from build123d import *
from OCP.BRepFilletAPI import BRepFilletAPI_MakeChamfer

# Parameters (mm, degrees)
CROQUIS1_W              = 16
CROQUIS1_H              = 65
CROQUIS1_W_2            = 60.56813556
CROQUIS1_H_2            = 14.096609531
SALIENTE_EXTRUIR1_DEPTH = 50
CROQUIS3_W              = 16
CROQUIS3_H              = 3
CROQUIS3_W_2            = 3.053388568
CROQUIS3_H_2            = 16.41437111
CROQUIS3_W_3            = 3.044949639
CROQUIS3_H_3            = 14.096609531
CROQUIS3_W_4            = 3.024386733
SALIENTE_EXTRUIR2_DEPTH = 18
CHAFL_N2_SIZE           = 3
CHAFL_N2_SIZE2          = 1.732050808
CHAFL_N3_SIZE           = 5.196152423
CHAFL_N3_SIZE_2         = 3


with BuildPart() as part:
    # Croquis1 → Saliente-Extruir1 (new body)
    with BuildSketch(Plane.XY):
        with BuildLine():
            Line((-85, 0), (-85, -65))
            ThreePointArc((-85, -65), (-79.142135624, -79.142135624), (-65, -85))
            Line((-65, -85), (65, -85))
            ThreePointArc((65, -85), (79.142135624, -79.142135624), (85, -65))
            Line((85, -65), (85, 0))
            ThreePointArc((85, 0), (0, 85), (-85, 0))
        make_face()
        with Locations((75, -31.476837664)):
            Rectangle(CROQUIS1_W, CROQUIS1_H, mode=Mode.SUBTRACT)
        with BuildLine():
            Line((-65, -65), (65, -65))
            Line((65, -65), (65, 0))
            ThreePointArc((65, 0), (0, 65), (-65, 0))
            Line((-65, 0), (-65, -65))
        make_face(mode=Mode.SUBTRACT)
        with Locations((-75, -31.476837664)):
            Rectangle(CROQUIS1_W, CROQUIS1_H, mode=Mode.SUBTRACT)
        with BuildLine():
            Line((3.510152615, 83.023277843), (3.510152615, 66.83939974))
            ThreePointArc((3.510152615, 66.83939974), (47.145709065, 47.509037517), (66.810483413, 4.023162336))
            Line((66.810483413, 4.023162336), (83, 4.023162336))
            ThreePointArc((83, 4.023162336), (58.576925397, 58.940051292), (3.510152615, 83.023277843))
        make_face(mode=Mode.SUBTRACT)
        with BuildLine():
            Line((-66.810483413, 4.023162336), (-83, 4.023162336))
            ThreePointArc((-83, 4.023162336), (-58.576925397, 58.940051292), (-3.510152615, 83.023277843))
            Line((-3.510152615, 83.023277843), (-3.510152615, 66.83939974))
            ThreePointArc((-3.510152615, 66.83939974), (-47.145709065, 47.509037517), (-66.810483413, 4.023162336))
        make_face(mode=Mode.SUBTRACT)
        with BuildLine():
            Line((-81.096609531, -66.976837664), (-34.71593222, -66.976837664))
            Line((-34.71593222, -66.976837664), (-34.71593222, -81.073447195))
            Line((-34.71593222, -81.073447195), (-67, -81.073447195))
            ThreePointArc((-67, -81.073447195), (-76.967808191, -76.944645855), (-81.096609531, -66.976837664))
        make_face(mode=Mode.SUBTRACT)
        with BuildLine():
            Line((67, -81.073447195), (34.71593222, -81.073447195))
            Line((34.71593222, -81.073447195), (34.71593222, -66.976837664))
            Line((34.71593222, -66.976837664), (81.096609531, -66.976837664))
            ThreePointArc((81.096609531, -66.976837664), (76.967808191, -76.944645855), (67, -81.073447195))
        make_face(mode=Mode.SUBTRACT)
        with Locations((0, -74.025142429)):
            Rectangle(CROQUIS1_W_2, CROQUIS1_H_2, mode=Mode.SUBTRACT)
    extrude(amount=SALIENTE_EXTRUIR1_DEPTH)

    # Croquis3 → Saliente-Extruir2 (add)
    with BuildSketch(Plane.XY.offset(40)):
        with Locations((-75, -0.476837664)):
            Rectangle(CROQUIS3_W, CROQUIS3_H)
        with Locations((-75, -62.476837664)):
            Rectangle(CROQUIS3_W, CROQUIS3_H)
        with Locations((75, -62.476837664)):
            Rectangle(CROQUIS3_W, CROQUIS3_H)
        with Locations((75, -0.476837664)):
            Rectangle(CROQUIS3_W, CROQUIS3_H)
        with Locations((-5.036846899, 74.816092288)):
            Rectangle(CROQUIS3_W_2, CROQUIS3_H_2)
        with Locations((5.036846899, 74.816092288)):
            Rectangle(CROQUIS3_W_2, CROQUIS3_H_2)
        with Locations((-28.761592961, -74.025142429)):
            Rectangle(CROQUIS3_W_3, CROQUIS3_H_3)
        with Locations((28.771874414, -74.025142429)):
            Rectangle(CROQUIS3_W_4, CROQUIS3_H_3)
    extrude(amount=SALIENTE_EXTRUIR2_DEPTH)

    # Chaflán2: one chamfer whose edges measure the first distance from different faces: ONE call of the kernel's chamfer builder (chamfer() names one face for all edges)
    chafl_n2_edges_1 = [part.edges().sort_by_distance(p)[0] for p in [
        (-75, 1.023162336, 58),
    ]]
    chafl_n2_side_1 = [part.faces().sort_by_distance(p)[0] for p in [
        (-75, 1.023162336, 54),
    ]]
    chafl_n2_edges_2 = [part.edges().sort_by_distance(p)[0] for p in [
        (-75, -63.976837664, 58),
    ]]
    chafl_n2_side_2 = [part.faces().sort_by_distance(p)[0] for p in [
        (-75, -63.976837664, 54),
    ]]
    chafl_n2_edges_3 = [part.edges().sort_by_distance(p)[0] for p in [
        (75, -63.976837664, 58),
    ]]
    chafl_n2_side_3 = [part.faces().sort_by_distance(p)[0] for p in [
        (75, -63.976837664, 54),
    ]]
    chafl_n2_edges_4 = [part.edges().sort_by_distance(p)[0] for p in [
        (75, 1.023162336, 58),
    ]]
    chafl_n2_side_4 = [part.faces().sort_by_distance(p)[0] for p in [
        (75, 1.023162336, 54),
    ]]
    chafl_n2_edges_5 = [part.edges().sort_by_distance(p)[0] for p in [
        (-3.510152615, 74.816092288, 58),
    ]]
    chafl_n2_side_5 = [part.faces().sort_by_distance(p)[0] for p in [
        (-3.510152615, 74.816092288, 54),
    ]]
    chafl_n2_edges_6 = [part.edges().sort_by_distance(p)[0] for p in [
        (3.510152615, 74.816092288, 58),
    ]]
    chafl_n2_side_6 = [part.faces().sort_by_distance(p)[0] for p in [
        (3.510152615, 74.816092288, 54),
    ]]
    chafl_n2_edges_7 = [part.edges().sort_by_distance(p)[0] for p in [
        (-30.28406778, -74.025142429, 58),
    ]]
    chafl_n2_side_7 = [part.faces().sort_by_distance(p)[0] for p in [
        (-30.28406778, -74.025142429, 54),
    ]]
    chafl_n2_edges_8 = [part.edges().sort_by_distance(p)[0] for p in [
        (30.28406778, -74.025142429, 58),
    ]]
    chafl_n2_side_8 = [part.faces().sort_by_distance(p)[0] for p in [
        (30.28406778, -74.025142429, 54),
    ]]
    chafl_n2 = BRepFilletAPI_MakeChamfer(part.part.solid().wrapped)
    for e in chafl_n2_edges_1:
        chafl_n2.Add(CHAFL_N2_SIZE, CHAFL_N2_SIZE2, e.wrapped, chafl_n2_side_1[0].wrapped)  # the first distance lies on this face
    for e in chafl_n2_edges_2:
        chafl_n2.Add(CHAFL_N2_SIZE, CHAFL_N2_SIZE2, e.wrapped, chafl_n2_side_2[0].wrapped)  # the first distance lies on this face
    for e in chafl_n2_edges_3:
        chafl_n2.Add(CHAFL_N2_SIZE, CHAFL_N2_SIZE2, e.wrapped, chafl_n2_side_3[0].wrapped)  # the first distance lies on this face
    for e in chafl_n2_edges_4:
        chafl_n2.Add(CHAFL_N2_SIZE, CHAFL_N2_SIZE2, e.wrapped, chafl_n2_side_4[0].wrapped)  # the first distance lies on this face
    for e in chafl_n2_edges_5:
        chafl_n2.Add(CHAFL_N2_SIZE, CHAFL_N2_SIZE2, e.wrapped, chafl_n2_side_5[0].wrapped)  # the first distance lies on this face
    for e in chafl_n2_edges_6:
        chafl_n2.Add(CHAFL_N2_SIZE, CHAFL_N2_SIZE2, e.wrapped, chafl_n2_side_6[0].wrapped)  # the first distance lies on this face
    for e in chafl_n2_edges_7:
        chafl_n2.Add(CHAFL_N2_SIZE, CHAFL_N2_SIZE2, e.wrapped, chafl_n2_side_7[0].wrapped)  # the first distance lies on this face
    for e in chafl_n2_edges_8:
        chafl_n2.Add(CHAFL_N2_SIZE, CHAFL_N2_SIZE2, e.wrapped, chafl_n2_side_8[0].wrapped)  # the first distance lies on this face
    add(Compound.cast(chafl_n2.Shape()), mode=Mode.REPLACE)

    # Chaflán3
    chafl_n3_edges_1 = [part.edges().sort_by_distance(p)[0] for p in [
        (75, -60.976837664, 40),
    ]]
    chafl_n3_side_1 = [part.faces().sort_by_distance(p)[0] for p in [
        (75, -60.976837664, 40.06),
    ]]
    chafl_n3_edges_2 = [part.edges().sort_by_distance(p)[0] for p in [
        (75, -1.976837664, 40),
    ]]
    chafl_n3_side_2 = [part.faces().sort_by_distance(p)[0] for p in [
        (75, -1.976837664, 40.06),
    ]]
    chafl_n3_edges_3 = [part.edges().sort_by_distance(p)[0] for p in [
        (27.259681047, -74.025142429, 40),
    ]]
    chafl_n3_side_3 = [part.faces().sort_by_distance(p)[0] for p in [
        (27.319681047, -74.025142429, 40),
    ]]
    chafl_n3_edges_4 = [part.edges().sort_by_distance(p)[0] for p in [
        (-27.239118141, -74.025142429, 40),
    ]]
    chafl_n3_side_4 = [part.faces().sort_by_distance(p)[0] for p in [
        (-27.239118141, -74.025142429, 40.06),
    ]]
    chafl_n3_edges_5 = [part.edges().sort_by_distance(p)[0] for p in [
        (-75, -60.976837664, 40),
    ]]
    chafl_n3_side_5 = [part.faces().sort_by_distance(p)[0] for p in [
        (-75, -60.976837664, 40.06),
    ]]
    chafl_n3_edges_6 = [part.edges().sort_by_distance(p)[0] for p in [
        (-75, -1.976837664, 40),
    ]]
    chafl_n3_side_6 = [part.faces().sort_by_distance(p)[0] for p in [
        (-75, -1.976837664, 40.06),
    ]]
    chafl_n3_edges_7 = [part.edges().sort_by_distance(p)[0] for p in [
        (-6.563541183, 74.72336741, 40),
    ]]
    chafl_n3_side_7 = [part.faces().sort_by_distance(p)[0] for p in [
        (-6.563541183, 74.72336741, 40.06),
    ]]
    chafl_n3_edges_8 = [part.edges().sort_by_distance(p)[0] for p in [
        (6.563541183, 74.72336741, 40),
    ]]
    chafl_n3_side_8 = [part.faces().sort_by_distance(p)[0] for p in [
        (6.563541183, 74.72336741, 40.06),
    ]]
    chafl_n3 = BRepFilletAPI_MakeChamfer(part.part.solid().wrapped)
    for e in chafl_n3_edges_1:
        chafl_n3.Add(CHAFL_N3_SIZE - 0.0001, CHAFL_N3_SIZE_2 - 0.0001, e.wrapped, chafl_n3_side_1[0].wrapped)
    for e in chafl_n3_edges_2:
        chafl_n3.Add(CHAFL_N3_SIZE - 0.0001, CHAFL_N3_SIZE_2 - 0.0001, e.wrapped, chafl_n3_side_2[0].wrapped)
    for e in chafl_n3_edges_3:
        chafl_n3.Add(CHAFL_N3_SIZE_2 - 0.0001, CHAFL_N3_SIZE - 0.0001, e.wrapped, chafl_n3_side_3[0].wrapped)
    for e in chafl_n3_edges_4:
        chafl_n3.Add(CHAFL_N3_SIZE - 0.0001, CHAFL_N3_SIZE_2 - 0.0001, e.wrapped, chafl_n3_side_4[0].wrapped)
    for e in chafl_n3_edges_5:
        chafl_n3.Add(CHAFL_N3_SIZE - 0.0001, CHAFL_N3_SIZE_2 - 0.0001, e.wrapped, chafl_n3_side_5[0].wrapped)
    for e in chafl_n3_edges_6:
        chafl_n3.Add(CHAFL_N3_SIZE - 0.0001, CHAFL_N3_SIZE_2 - 0.0001, e.wrapped, chafl_n3_side_6[0].wrapped)
    for e in chafl_n3_edges_7:
        chafl_n3.Add(CHAFL_N3_SIZE - 0.0001, CHAFL_N3_SIZE_2 - 0.0001, e.wrapped, chafl_n3_side_7[0].wrapped)
    for e in chafl_n3_edges_8:
        chafl_n3.Add(CHAFL_N3_SIZE - 0.0001, CHAFL_N3_SIZE_2 - 0.0001, e.wrapped, chafl_n3_side_8[0].wrapped)
    add(Compound.cast(chafl_n3.Shape()), mode=Mode.REPLACE)  # a hair under: the kernel refuses the full size


solid = part.part
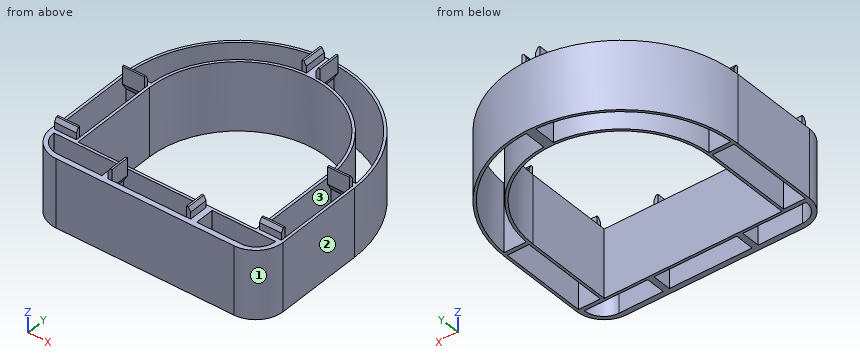
Source: CAD feature listing. Evaluate the final solid. Frame: model axes, mm. Face numbers are marked on the shaded views. Round coordinates to 2 decimals unless told otherwise and drop trailing zeros. Loops run counter-clockwise (first coordinate to the right, second up) from the corner with the lowest first, then second, coordinate; pieces in that order, holes last. Notation, with made-up numbers: M 79.5,-23.5 L 83.5,-23.5 A25 ccw 83.5,-9.5 Z; hole C 8,23 d10. An arc over 180 degrees is marked long. Return JSON: item names as keys, results as strings. Group by question number.
1. Section query B-B on y = -54. Output: boundary loops of the cut face in (x, z), and give its area (3 significant figures).
2. Pin query (flat end, axial travel): pin 1 (15.5 mm diameter, centred on y = -75.5, z = 23, fed in from -X); pin 2 (1.5 mm diameter, centred on x = -64.5, z = 36.5, fed in from +Y); pin 3 (0.9 mm diameter, centred on x = -4.5, z = 54.5, fed in from +Y); pin 4 (12 mm diameter, centred on x = -29.5, y = 55, fed in from -Z). Return the tip coordinate at first contact, or that it passes through.
3. Section query D-D on x = -45.5. Output: boundary loops of the cut face in (y, z).
4. Section query C-C on x = 0. Output: boundary loops of the cut face in (y, z), and give its area (3 significant figures).
5. Material intervals for line 1 along X through (y, z) = (-27.5, 11); line 2 along Y through (x, z) = (-8.5, 18); line 3 along Y through (x, z) = (11.5, 44.5), sorted ascending. Write a range as from..to.
6. Section query A-A on z = 52. State how many separate pieces and enclosed holes the cut face has, and give its area (3 significant figures).
7. Mould query, pull axis Y, two halves, no side actions, for the marked faces 1, 2 and 3. Classes: released by +Y, released by -Y, zero draft, split by the parting line, or undercut.
Checks:
{
 "1": {"outline": "M -85,0 L -83,0 L -83,50 L -85,50 Z; M -67,0 L -65,0 L -65,50 L -67,50 Z; M 65,0 L 67,0 L 67,50 L 65,50 Z; M 83,0 L 85,0 L 85,50 L 83,50 Z", "area": "400 mm²"},
 "2": {"pin 1": "stops at x = -84.81", "pin 2": "stops at y = 56.22", "pin 3": "stops at y = 83.02", "pin 4": "stops at z = 0"},
 "3": {"outline": "M -85,0 L -81.07,0 L -81.07,50 L -85,50 Z; M -66.98,0 L -65,0 L -65,50 L -66.98,50 Z; M 46.42,0 L 49.09,0 L 49.09,50 L 46.42,50 Z; M 69.53,0 L 71.8,0 L 71.8,50 L 69.53,50 Z"},
 "4": {"outline": "M -85,0 L -81.07,0 L -81.07,50 L -85,50 Z; M -66.98,0 L -65,0 L -65,50 L -66.98,50 Z; M 65,0 L 85,0 L 85,50 L 65,50 Z", "area": "1,300 mm²"},
 "5": {"line 1": "x = -85..-83, -67..-65, 65..67, 83..85", "line 2": "y = -85..-81.07, -66.98..-65, 64.44..66.39, 82.66..84.57", "line 3": "y = -85..-81.07, -66.98..-65, 63.97..65.94, 82.3..84.22"},
 "6": {"separate pieces": "8", "enclosed holes": "0", "area": "378 mm²"},
 "7": {"face 1": "released by -Y", "face 2": "zero draft", "face 3": "undercut"}
}
